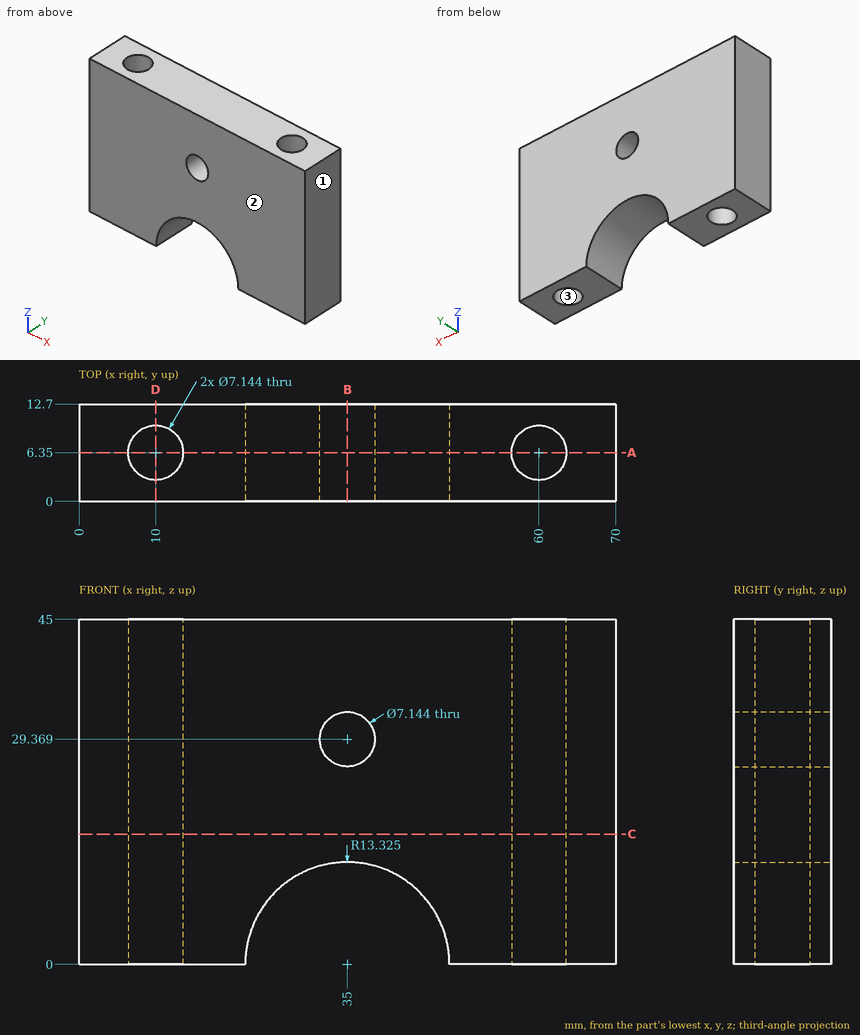
Study the drawing (mm; zero at the part's minimum x, y, z) and answer. Give positions to 0.01 mm unless a question says otherwise; leave off trailing zeros. Write each loop counter-clockwise with the first axis right and the second up, starting at its lowest first coordinate (ties: lowest second). Pieces come first, ordered by that corner, then holes.
(1) The part is cut by section A-A on y = 6.35. Count the separate pieces of the cut face and the enclosed holes in it, plus the area to 3 significant figures.
Final values:
separate pieces: 3
enclosed holes: 1
area: 2,190 mm2
(2) The mould has two halves that part along Y. Classify the marked faces 1, 2 and 3: pulls with the +Y half, pulls with the -Y half, needs draft (parallel to the pull), parting line crosses it, or undercut.
Final values:
face 1: needs draft
face 2: pulls with the -Y half
face 3: undercut
(3) The part is cut by section B-B on x = 35. Write down the section's boundary in (y, z) (1 decimal).
Final values:
outline: (0, 13.3) - (12.7, 13.3) - (12.7, 25.8) - (0, 25.8) - close; (0, 32.9) - (12.7, 32.9) - (12.7, 45) - (0, 45) - close
(4) Straight lines are drawn through the part: line 1 (X direction, y = 6.35, z = 20); line 2 (Z direction, x = 35, y = 6.25) (1 decimal); line 3 (X direction, y = 8.5, z = 36.5). For each, find the intervals that lie inside material, in ascending order.
Final values:
line 1: x = 0 to 6.43, 13.57 to 56.43, 63.57 to 70
line 2: z = 13.3 to 25.8, 32.9 to 45
line 3: x = 0 to 7.15, 12.85 to 57.15, 62.85 to 70
(5) A flat-ended cylindrical pin translates along its axis: pin 1 Ø2 at (x, y) = (33, 4) entering from -Z. Find the tip coordinate at first contact, or state that the pin passes through.
Final values:
pin 1: stops at z = 12.98
(6) The part is cut by section C-C on z = 17. Write down the section's boundary in (x, y).
Final values:
outline: (0, 0) - (70, 0) - (70, 12.7) - (0, 12.7) - close; hole circle Ø7.14 at (10, 6.35); hole circle Ø7.14 at (60, 6.35)
(7) The part is cut by section D-D on x = 10. Write down the section's boundary in (y, z), plus the area to 3 significant figures.
Final values:
outline: (0, 0) - (2.78, 0) - (2.78, 45) - (0, 45) - close; (9.92, 0) - (12.7, 0) - (12.7, 45) - (9.92, 45) - close
area: 250 mm2
